Job drawing, mm, ordinate dimensions from the low corner. One solid piece. Give positions to 0.01 mm unless a question says otherwise; leave off trailing zeros. Write each loop counter-clockwise with the first axis right and the second up, starting at its lowest first coordinate (ties: lowest second). Pieces come first, ordered by that corner, then holes. Notation, with made-up numbers: (-6, 47) - (31, 47) arc R32 ccw to (31, 79) - close; hole circle Ø7 at (60.5, 24.5). An arc over 180 degrees is marked (long way). Answer in a Markdown table with one row per item. Add a question column.
1. Band-saw the part on C-C on z = 28.5. Write the cut outline in (x, y).
2. Probe line 1 along Z through (x, y) = (60.5, 3.25) (1 decimal); line 2 along X through (y, z) = (1.75, 95) (1 decimal); line 3 along X through (y, z) = (23.75, 32) (1 decimal). List the from-to ranges inside material, lowest first.
3. Drop flat-ended pins along their axis: pin 1 Ø5.5 at (x, z) = (62.75, 78.34) entering from +Y; pin 2 Ø12 at (y, z) = (15.5, 78.5) entering from +X; pin 3 Ø1.5 at (y, z) = (5.5, 55) entering from +X; pin 4 Ø6 at (x, y) = (13.5, 9) entering from -Z (1 decimal). Give the stop position or say it passes through.
4. Band-saw the part on B-B on x = 47. Write the cut outline in (y, z) (1 decimal), plus the area to 3 significant figures.
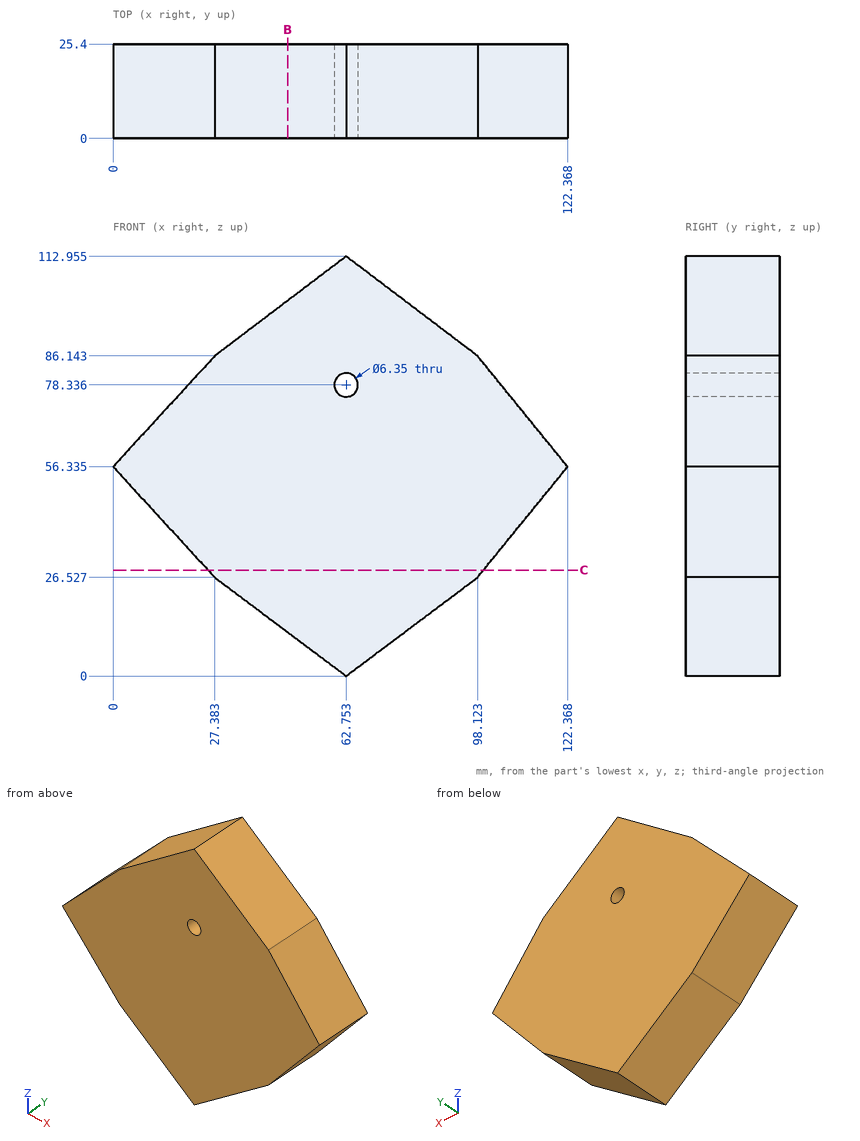
Values:
| question | item | result |
|---|---|---|
| 1 | outline | (25.57, 0) - (99.73, 0) - (99.73, 25.4) - (25.57, 25.4) - close |
| 2 | line 1 | z = 1.7 to 76.1, 80.6 to 111.2 |
| 2 | line 2 | x = 39.1 to 86.4 |
| 2 | line 3 | x = 22.4 to 102.6 |
| 3 | pin 1 | passes through |
| 3 | pin 2 | stops at x = 109.22 |
| 3 | pin 3 | stops at x = 121.89 |
| 3 | pin 4 | stops at z = 38.4 |
| 4 | outline | (0, 11.8) - (25.4, 11.8) - (25.4, 101) - (0, 101) - close |
| 4 | area | 2,270 mm² |
